Autodesk Inventor part; units mm, degrees
ref_plane "YZ Plane" through (0, 0, 0) normal (1, 0, 0) x (0, 1, 0)
ref_plane "XZ Plane" through (0, 0, 0) normal (0, 1, 0) x (-1, 0, 0)
ref_plane "XY Plane" through (0, 0, 0) normal (0, 0, 1) x (1, 0, 0)
sketch "Эскиз1" plane through (0, 0, 0) normal (0, 1, 0) x (-1, 0, 0)
  line L0 (-42.5, 221) -> (42.5, 221)
  line L1 (42.5, 221) -> (42.5, -221)
  line L2 (42.5, -221) -> (-42.5, -221)
  line L3 (-42.5, -221) -> (-42.5, 221)
  line L4 (-42.5, 221) -> (42.5, -221) construction
  line L5 (42.5, 221) -> (-42.5, -221) construction
  line L6 (-42.5, 140) -> (-42.5, 50)
  line L7 (-42.5, 50) -> (-46.5, 50)
  line L8 (-46.5, 50) -> (-46.5, 140)
  line L9 (-46.5, 140) -> (-42.5, 140)
  line L10 (0, 0) -> (-15, 0) construction
  line L11 (-46.5, -50) -> (-46.5, -140)
  line L12 (-46.5, -140) -> (-42.5, -140)
  line L13 (-42.5, -50) -> (-46.5, -50)
  line L14 (-42.5, -140) -> (-42.5, -50)
  line L15 (-42.5, -24) -> (-42.5, 66)
  line L16 (15, 225) -> (15, 221)
  line L17 (15, 221) -> (-15, 221)
  line L18 (-15, 221) -> (-15, 225)
  line L19 (-15, 225) -> (15, 225)
  line L20 (15, 225) -> (-15, 221) construction
  line L21 (15, 221) -> (-15, 225) construction
  line L22 (0, 0) -> (0, 26.5579) construction
  line L23 (15, -225) -> (15, -221)
  line L24 (15, -221) -> (-15, -221)
  line L25 (-15, -221) -> (-15, -225)
  line L26 (-15, -225) -> (15, -225)
  point P0 (-10, -165.5)
  point P1 (-10, -255.5)
  point P2 (-10, -45)
  point P3 (-10, 45)
  point P4 (-42.5, -50)
  point P5 (-42.5, -140)
  point P6 (0, 223)
  point P7 (0, 223)
  point P8 (-15, -221)
  point P9 (15, -221)
  dimension "d0" = 442
  dimension "d1" = 85
  dimension "d2" = 4
  dimension "d3" = 90
  dimension "d4" = 50
  dimension "d9" = 30
  dimension "d11" = 4
extrude "Выдавливание1" add sketch "Эскиз1" along normal blind 4
properties part number "стенка боковая"
Model file for the job. Use its own axes, mm. Give positions to 0.01 mm unless a question says otherwise; leave off trailing zeros. Order: outer loops, then holes, each group sorted by start corner. A loop starts at its lowest first (then second) coordinate and runs counter-clockwise, first axis right, second up. Notation, with made-up numbers: (11.5, 78.25) -> (31.5, 78.25) arc R14 cw to (31.5, 82.25) -> close; hole circle Ø8 at (-29, 39). An arc over 180 degrees is marked (long way). Use CSV: the item, a comma, the result in double quotes.
1. Drill centre lines: line 1 along X through (y, z) = (2.15, 30); line 2 along Z through (x, y) = (-24, 0.65). Where is each one in solid material? Low to high. Write a range as from..to.
Outcome:
line 1,"-42.5..42.5"
line 2,"-221..221"
2. Band-saw the part on C-C, the plane z = -9. Give the cut face in (x, y), then the cut area to 3 significant figures.
Outcome:
outline,"(-42.5, 0) -> (42.5, 0) -> (42.5, 4) -> (-42.5, 4) -> close"
area,"340 mm²"
3. Band-saw the part on B-B, the plane x = -26.5. Give the cut face in (y, z), then the cut area to 3 significant figures.
Outcome:
outline,"(0, -221) -> (4, -221) -> (4, 221) -> (0, 221) -> close"
area,"1,770 mm²"
4. Drop flat-ended pins along their axis: pin 1 (1.2 mm diameter, centred on x = 44.5, y = 2, fed in from +Z); pin 2 (2 mm diameter, centred on x = -27, y = 1, fed in from +Z); pin 3 (1.2 mm diameter, centred on x = 31, y = 2.5, fed in from -Z). Give the stop position or say it passes through.
Outcome:
pin 1,"z = 140"
pin 2,"z = 221"
pin 3,"z = -221"
5. Band-saw the part on A-A, the plane y = 2.85. Give the cut face in (x, z).
Outcome:
outline,"(-42.5, -221) -> (-15, -221) -> (-15, -225) -> (15, -225) -> (15, -221) -> (42.5, -221) -> (42.5, -140) -> (46.5, -140) -> (46.5, -50) -> (42.5, -50) -> (42.5, 50) -> (46.5, 50) -> (46.5, 140) -> (42.5, 140) -> (42.5, 221) -> (15, 221) -> (15, 225) -> (-15, 225) -> (-15, 221) -> (-42.5, 221) -> close"
